```python
from build123d import *

# Parameters (mm, degrees)
SKETCH1_R          = 3.2512
SKETCH1_R_2        = 1.3462
EXTRUDE1_DEPTH     = 0.6223
SKETCH2_R          = 2.2987
CUT_EXTRUDE1_DEPTH = 0.37338
CUT_EXTRUDE2_DEPTH = 1.87122
CIRPATTERN1_COUNT  = 2


with BuildPart() as part:
    # Sketch1 → Extrude1 (new body, symmetric)
    with BuildSketch(Plane.XY):
        Circle(SKETCH1_R)
        Circle(SKETCH1_R_2, mode=Mode.SUBTRACT)
    extrude(amount=EXTRUDE1_DEPTH, both=True)

    # Sketch2 → Cut-Extrude1 (cut)
    with BuildSketch(Plane.XY.offset(0.6223)):
        Circle(SKETCH2_R)
    extrude(amount=-CUT_EXTRUDE1_DEPTH, mode=Mode.SUBTRACT)

    # Sketch3 → Cut-Extrude2 (cut, through all)
    with BuildSketch(Plane.XY.offset(0.24892)):
        with BuildLine():
            Line((-1.00965, 2.065097714), (-1.00965, 0.890427604))
            ThreePointArc((-1.00965, 0.890427604), (0, 1.3462), (1.00965, 0.890427604))
            Line((1.00965, 0.890427604), (1.00965, 2.065097714))
            ThreePointArc((1.00965, 2.065097714), (0, 2.2987), (-1.00965, 2.065097714))
        make_face()
    cut_extrude2 = extrude(amount=-CUT_EXTRUDE2_DEPTH, mode=Mode.SUBTRACT)

    # CirPattern1: Cut-Extrude2 ×2 about axis
    cirpattern1_axis = Axis((0, 0, 0.6223), (0, 0, -1))
    for i in range(1, CIRPATTERN1_COUNT):
        add(cut_extrude2.rotate(cirpattern1_axis, i * 360 / CIRPATTERN1_COUNT), mode=Mode.SUBTRACT)


solid = part.part
```
Geometry check sheet. Reference: the model listing, model coordinates, mm. A direction names the side the tool comes from. Round coordinates to 2 decimals unless told otherwise and drop trailing zeros. Loops run counter-clockwise (first coordinate to the right, second up) from the corner with the lowest first, then second, coordinate; pieces in that order, holes last. Notation, with made-up numbers: (85.25, 76.5) - (105.25, 76.5) arc R15 ccw to (105.25, 99.5) - close; hole circle Ø6 at (-21.5, 56.5). An arc over 180 degrees is marked (long way). Write each question's results on one line, items separated by ' | '. Start each with the question number.
Q1. Cross-section at B-B on y = 0. Enter the section's corners in (x, z), and give its area (3 significant figures).
Q2. Cross-section at C-C on z = -0.45. Enter the section's corners in (x, y).
Q3. Access from +Z, -Z, +X, -X, +Y, -Y to the whole of each face (thin tool, end or side, straight path). Record for faces 5 (the flat face through (-2, 0, 0.249)), 6 (the flat face through (-1.01, 1.5, -0.2)), 7 (the flat face through (1.4, -2.1, 0.622)).
Q4. Thickness scan on line 1 (Y direction, x = 0, z = 0.55); line 2 (X direction, y = 1.5, z = -0.3); line 3 (Z direction, x = 1.25, y = 1). Record the ranges inside material, lowest first. Write a range as [from, to].
Q5. Release check for a two-part mould opening along Y. For faces 1 (the flat face through (2, 0, 0.249)), 2 (the cylindrical face through (-1.346, 0.014, -0.193)), 3 (the flat face through (1.4, -0.7, -0.622)), 4 (the cylindrical face through (-0.423, 3.224, 0.009)) record: +Y half, -Y half, draft (parallel to the pull), parting line (faces both ways), or undercut.
Q6. Cross-section at A-A on x = 0. Enter the section's corners in (y, z), and give its area (3 significant figures).
Q7. Gauge pin test, flat ends, axial feed: P1, Ø0.7, axis at y = 1.5, z = -0.5, coming from the -X side; P2, Ø0.6, axis at x = 1.5, y = -1, coming from the +Z side. Record the tip position at first contact, or that the pin passes through.
Q8. Cross-section at D-D on x = -1.5. Enter the section's corners in (y, z).
Answers below:
1) outline: (-3.25, -0.62) - (-1.35, -0.62) - (-1.35, 0.25) - (-2.3, 0.25) - (-2.3, 0.62) - (-3.25, 0.62) - close; (1.35, -0.62) - (3.25, -0.62) - (3.25, 0.62) - (2.3, 0.62) - (2.3, 0.25) - (1.35, 0.25) - close | area: 4.03 mm²
2) outline: circle Ø6.5 at (0, 0); hole (-1.01, -2.07) arc R2.3 ccw to (1.01, -2.07) - (1.01, -0.89) arc R1.35 ccw to (1.01, 0.89) - (1.01, 2.07) arc R2.3 ccw to (-1.01, 2.07) - (-1.01, 0.89) arc R1.35 ccw to (-1.01, -0.89) - close
3) face 5: +Z | face 6: +Z, -Z | face 7: +Z, +X, -X, +Y, -Y
4) line 1: y = [-3.25, -2.3], [2.3, 3.25] | line 2: x = [-2.88, -1.01], [1.01, 2.88] | line 3: z = [-0.62, 0.25]
5) face 1: undercut | face 2: undercut | face 3: draft | face 4: parting line
6) outline: (-3.25, -0.62) - (-2.3, -0.62) - (-2.3, 0.62) - (-3.25, 0.62) - close; (2.3, -0.62) - (3.25, -0.62) - (3.25, 0.62) - (2.3, 0.62) - close | area: 2.37 mm²
7) P1: stops at x = -3.04 | P2: stops at z = 0.25
8) outline: (-2.88, -0.62) - (2.88, -0.62) - (2.88, 0.62) - (1.74, 0.62) - (1.74, 0.25) - (-1.74, 0.25) - (-1.74, 0.62) - (-2.88, 0.62) - close
